Input: part model. Units: mm. Frame: model coordinates. A direction names the side the tool comes from. Coordinates: 2 decimals unless noted, no trailing zeros. Loops run counter-clockwise (first coordinate to the right, second up) from the corner with the lowest first, then second, coordinate; pieces in that order, holes last. Notation, with made-up numbers: (43.25, 49.25) -> (71.25, 49.25) arc R21 cw to (71.25, 63.25) -> close; hole circle Ø7 at (10.5, -17.75). An arc over 180 degrees is marked (long way). Put each result on its own line as item: value. Start each with the question number.
1) Material intervals for L1, parallel to Z at x = 0, y = 17.35 (1 decimal); L2, parallel to Y at x = 1, z = -2; L3, parallel to Y at x = 3.5, z = 11, sorted ascending.
2) Set-up query: faces 5 (the flat face through (0, 8, -11.5)), 6 (the flat face through (0, 0, 0)), 7 (the flat face through (0, 18.2, 15)), 8 (the flat face through (0, 18.2, -15)), 9 (the flat face through (0, 26.7, 2)). Return all of +Z, -Z, +X, -X, +Y, -Y with unobstructed straight access to the full face (end or side cutting, diameter ignored); none if empty.
3) Cut plane C-C (y = 17.75). Return the cut outline in (x, z) (1 decimal), plus the area to 3 significant figures.
4) Pull-direction query (Z, two-part tool) for faces 1 (the flat face through (0, 20, 11.5)), 2 (the flat face through (0, 15.7, 15)), 3 (the flat face through (0, 17, -16.125)), 4 (the cylindrical face through (-0.07, 24.47, -3.35)); classes: pulls with the +Z half, pulls with the -Z half, needs draft (parallel to the pull), parting line crosses it, or undercut.
5) Contact query for flat-ended pins moving along their axis: P1, Ø3.5, axis at x = 3, z = 0.5, coming from the +Y side; P2, Ø6, axis at x = -1, y = 6, coming from the +Z side; P3, Ø5, axis at x = -1.5, z = -13.5, coming from the +Y side. Output: stop coordinate, or through.
6) Cut plane B-B (z = 5.5). Return the cut outline in (x, y) (3 decimals), plus the area to 3 significant figures.
7) Cut plane A-A (x = 0). State how many separate pieces and enclosed holes the cut face has, plus the area to 3 significant figures.
8) Cut plane D-D (y = 11.25). Return the cut outline in (x, z), plus the area to 3 significant figures.
Autodesk Inventor part; units mm, degrees
ref_plane "Work Plane1" through (0, 18.2, 0) normal (0, -1, 0) x (1, 0, 0)
ref_plane "Work Plane2" through (-6, 0, 0) normal (0, 0, 1) x (1, 0, 0)
ref_plane "YZ Plane" through (0, 0, 0) normal (1, 0, 0) x (0, 1, 0)
sketch "Sketch1" plane through (0, 0, 0) normal (0, 1, 0) x (-1, 0, 0)
  line L0 (-6, 11.5) -> (6, 11.5)
  line L1 (6, 11.5) -> (6, -11.5)
  line L2 (6, -11.5) -> (-6, -11.5)
  line L3 (-6, -11.5) -> (-6, 11.5)
  point P0 (0, 0)
  point P1 (6, 0)
  point P2 (0, -11.5)
  dimension "d0" = 12
  dimension "d1" = 23
  dimension "d2" = 0
  dimension "d3" = 0
extrude "Extrusion1" add sketch "Sketch1" along normal blind 22.3
ref_plane "Work Plane1" through (0, 18.2, 0) normal (0, -1, 0) x (1, 0, 0)
sketch "Sketch2" plane through (0, 18.2, 0) normal (0, -1, 0) x (1, 0, 0)
  line L0 (-6, -11.5) -> (-6, 11.5)
  line L1 (-6, 11.5) -> (6, 11.5)
  line L2 (6, 11.5) -> (6, 16.125)
  line L3 (6, 16.125) -> (-6, 16.125)
  line L4 (-6, 16.125) -> (-6, 11.5)
  circle A0 centre (0, 13.8125) radius 1
  point P0 (0, 0)
  point P1 (0, 16.125)
  point P2 (6, 13.8125)
  dimension "d7" = 12
  dimension "d8" = 4.625
  dimension "d9" = 2
  dimension "d10" = 0
  dimension "d11" = 0
extrude "Extrusion2" add sketch "Sketch2" along normal blind 2.5
ref_plane "Work Plane2" through (-6, 0, 0) normal (0, 0, 1) x (1, 0, 0)
mirror "Mirror1" about plane through (-6, 0, 0) normal (0, 0, 1) of "Extrusion2"
sketch "Sketch3" plane through (0, 22.3, 0) normal (0, 1, 0) x (1, 0, 0)
  line L0 (6, 11.5) -> (-6, 11.5)
  line L1 (-6, 11.5) -> (-6, -11.5)
  line L2 (-6, -11.5) -> (6, -11.5)
  line L3 (6, -11.5) -> (6, 11.5)
  circle A0 centre (0, -5.5) radius 5.85
  circle A1 centre (0, 0.55) radius 2.8
  point P0 (0, 0)
  point P1 (0, -11.5)
  point P2 (2.6696, -0.2946)
  point P3 (-2.6696, -0.2946)
  dimension "d16" = 11.7
  dimension "d17" = 0
  dimension "d18" = 6
  dimension "d21" = 5.6
  dimension "d22" = 0
  dimension "d23" = 6.05
extrude "Extrusion3" add sketch "Sketch3" along normal blind 4.4 contours A0 A1 | A1 A0 | A0 A1
sketch "Sketch4" plane through (0, 26.7, 0) normal (0, 1, 0) x (1, 0, 0)
  arc A0 (-2.6696, -0.2946) -> (2.6696, -0.2946) centre (0, -5.5) ccw
  arc A1 (2.6696, -0.2946) -> (-2.6696, -0.2946) centre (0, 0.55) ccw
  circle A2 centre (0, -5.5) radius 2.375
  point P0 (0, 0)
  dimension "d24" = 4.75
extrude "Extrusion4" add sketch "Sketch4" along normal blind 3 contours A2
properties part number "Servo Motor"
Results found:
1. L1: z = -16.1 to -14.8, -12.8 to 12.8, 14.8 to 16.1
1. L2: y = 0 to 26.7
1. L3: y = 0 to 22.3
2. face 5: -Z, +X, -X, -Y
2. face 6: +Z, -Z, +X, -X, -Y
2. face 7: +Z, +X, -X, +Y
2. face 8: -Z, +X, -X, +Y
2. face 9: +Y
3. outline: (-6, -16.1) -> (6, -16.1) -> (6, 16.1) -> (-6, 16.1) -> close; hole circle Ø2 at (0, -13.8); hole circle Ø2 at (0, 13.8)
3. area: 381 mm2
4. face 1: pulls with the +Z half
4. face 2: needs draft
4. face 3: pulls with the -Z half
4. face 4: undercut
5. P1: stops at y = 26.7
5. P2: stops at z = 11.5
5. P3: stops at y = 22.3
6. outline: (-6, 0) -> (6, 0) -> (6, 22.3) -> (5.85, 22.3) -> (5.85, 26.7) -> (2.375, 26.7) -> (2.375, 29.7) -> (-2.375, 29.7) -> (-2.375, 26.7) -> (-5.85, 26.7) -> (-5.85, 22.3) -> (-6, 22.3) -> close
6. area: 333 mm2
7. separate pieces: 3
7. enclosed holes: 0
7. area: 605 mm2
8. outline: (-6, -11.5) -> (6, -11.5) -> (6, 11.5) -> (-6, 11.5) -> close
8. area: 276 mm2
